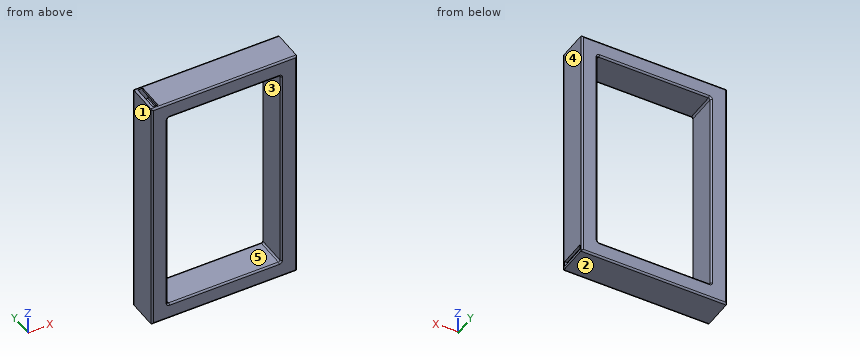
from build123d import *

# Parameters (mm, degrees)
F1_W     = 101.6
F1_H     = 50.8
F1_W_2   = 82.55
F1_H_2   = 34.8846255165
F4_W     = 50.8
F4_H     = 101.6
F4_W_2   = 31.75
F4_H_2   = 82.55
F6_DEPTH = 50.8
F7_F1_R  = 5.08
F7_F2_R  = 5.08
F8_R     = 5.08


with BuildPart() as f2:
    # F2: sweep along a path in F0
    with BuildLine(Plane.XZ) as f2_path:
        Line((0, 0), (406.4, 0))
        Line((406.4, 0), (406.4, -711.2))
    # F1 (on Right) → F2 (sweep)
    with BuildSketch(Plane.YZ):
        Rectangle(F1_W, F1_H)
        Rectangle(F1_W_2, F1_H_2, mode=Mode.SUBTRACT)
    sweep(path=f2_path.line, transition=Transition.RIGHT)

    # F5: sweep along a path in F0
    with BuildLine(Plane.XZ) as f5_path:
        Line((0, 0), (0, -711.2))
        Line((0, -711.2), (406.4, -711.2))
    # F4 (on offset) → F5 (sweep)
    with BuildSketch(Plane.XY.offset(25.4)):
        Rectangle(F4_W, F4_H)
        Rectangle(F4_W_2, F4_H_2, mode=Mode.SUBTRACT)
    sweep(path=f5_path.line, transition=Transition.RIGHT)

    # F6 (add): a face of the model
    f6_faces = [f2.faces().sort_by_distance(p)[0] for p in [
        (381, 0, -728.8136904762),
    ]]
    extrude(f6_faces, amount=F6_DEPTH)

    # F7: fillet of radius 5.08 on 6 edges, made by hand

    # F7_f1
    f7_f1_edges = [f2.edges().sort_by_distance(p)[0] for p in [
        (381, 0, -685.8),
        (25.4, 0, -685.8),
        (25.4, 0, -25.4),
        (381, 0, -25.4),
    ]]
    fillet(f7_f1_edges, radius=F7_F1_R)

    # F7_f2
    f7_f2_edges = [f2.edges().sort_by_distance(p)[0] for p in [
        (203.2, -50.8, -25.4),
        (25.4, 50.8, -355.6),
        (26.8878975516, 50.8, -26.8878975516),
        (26.8878975516, 50.8, -684.3121024484),
        (26.8878975516, -50.8, -26.8878975516),
        (379.5121024484, -50.8, -26.8878975516),
    ]]
    fillet(f7_f2_edges, radius=F7_F2_R)

    # F8
    f8_edges = [f2.edges().sort_by_distance(p)[0] for p in [
        (203.2, -50.8, 25.4),
        (-25.4, -50.8, -355.6),
        (431.8, -50.8, -355.6),
        (203.2, -50.8, -736.6),
        (-25.4, 50.8, -355.6),
        (203.2, 50.8, -736.6),
        (431.8, 50.8, -355.6),
        (203.2, 50.8, 25.4),
    ]]
    fillet(f8_edges, radius=F8_R)


solid = f2.part
For this review, take the finished solid that the model builds, in its own axes (mm). Face numbers are marked on the shaded views. A direction names the side the tool comes from. Give positions to 0.01 mm unless a question says otherwise; leave off trailing zeros. Order: outer loops, then holes, each group sorted by start corner. A loop starts at its lowest first (then second) coordinate and runs counter-clockwise, first axis right, second up. Notation, with made-up numbers: (-9.5, 89) - (18.5, 89) arc R22 cw to (18.5, 111) - close; hole circle Ø4 at (-2.75, 79). An arc over 180 degrees is marked (long way). Answer as a JSON object with one key per item and string values. Group by question number.
Item 1: Machinability: for the marked faces 4 and 5, which of the approach directions +Z, -Z, +X, -X, +Y, -Y give a long, thin tool a straight path to every point of the face, cutting with its end or side? Answer none if there is none.
Item 2: Draft analysis for pull direction X (two halves, no side actions). For the marked faces 1, 2 and 3, state which applies: pulls with the +X half, pulls with the -X half, needs draft (parallel to the pull), parting line crosses it, or undercut.
Item 3: Take a section at A-A on x = 336.5. Give the boundary of the cut face in (y, z) (3 decimals), and give its area (3 significant figures).
Item 4: Take a section at B-B on y = 24. Give the number of separate pieces and of enclosed holes in the cut face, and give its area (3 significant figures).
Item 5: Take a section at C-C on z = -215.5. Give the boundary of the cut face in (x, y) (3 decimals), and give its area (3 significant figures).
Item 6: Wall thickness on line 1 along X through (y, z) = (28.5, -421) (3 decimals); line 2 along Z through (x, y) = (213, 14.5) (3 decimals); line 3 along Z through (x, y) = (11.5, 9.5) (3 decimals): over which ranges is each line inside the solid? List them lowest first.
Reported:
{
 "1": {"face 4": "+Z, -Z, +X, +Y, -Y", "face 5": "+Y, -Y"},
 "2": {"face 1": "pulls with the -X half", "face 2": "needs draft", "face 3": "undercut"},
 "3": {"outline": "(-50.8, -731.52) arc R5.08 ccw to (-45.72, -736.6) - (45.72, -736.6) arc R5.08 ccw to (50.8, -731.52) - (50.8, -690.88) arc R5.08 ccw to (45.72, -685.8) - (-45.72, -685.8) arc R5.08 ccw to (-50.8, -690.88) - close; (-50.8, -20.32) arc R5.08 ccw to (-45.72, -25.4) - (45.72, -25.4) arc R5.08 ccw to (50.8, -20.32) - (50.8, 20.32) arc R5.08 ccw to (45.72, 25.4) - (-45.72, 25.4) arc R5.08 ccw to (-50.8, 20.32) - close; hole (-41.275, -727.075) - (41.275, -727.075) - (41.275, -695.325) - (-41.275, -695.325) - close; hole (-41.275, -17.442) - (41.275, -17.442) - (41.275, 17.442) - (-41.275, 17.442) - close", "area": "4,780 mm^2"},
 "4": {"separate pieces": "2", "enclosed holes": "1", "area": "39,400 mm^2"},
 "5": {"outline": "(-25.4, -45.72) arc R5.08 ccw to (-20.32, -50.8) - (20.32, -50.8) arc R5.08 ccw to (25.4, -45.72) - (25.4, 45.72) arc R5.08 ccw to (20.32, 50.8) - (-20.32, 50.8) arc R5.08 ccw to (-25.4, 45.72) - close; (381, -45.72) arc R5.08 ccw to (386.08, -50.8) - (426.72, -50.8) arc R5.08 ccw to (431.8, -45.72) - (431.8, 45.72) arc R5.08 ccw to (426.72, 50.8) - (386.08, 50.8) arc R5.08 ccw to (381, 45.72) - close; hole (-15.875, -41.275) - (15.875, -41.275) - (15.875, 41.275) - (-15.875, 41.275) - close; hole (388.958, -41.275) - (423.842, -41.275) - (423.842, 41.275) - (388.958, 41.275) - close", "area": "4,780 mm^2"},
 "6": {"line 1": "-25.4 to -15.875, 15.875 to 25.4, 381 to 388.958, 423.842 to 431.8", "line 2": "-736.6 to -727.075, -695.325 to -685.8, -25.4 to -17.442, 17.442 to 25.4", "line 3": "-736.6 to -727.075, -25.4 to -17.442, 17.442 to 25.4"}
}
